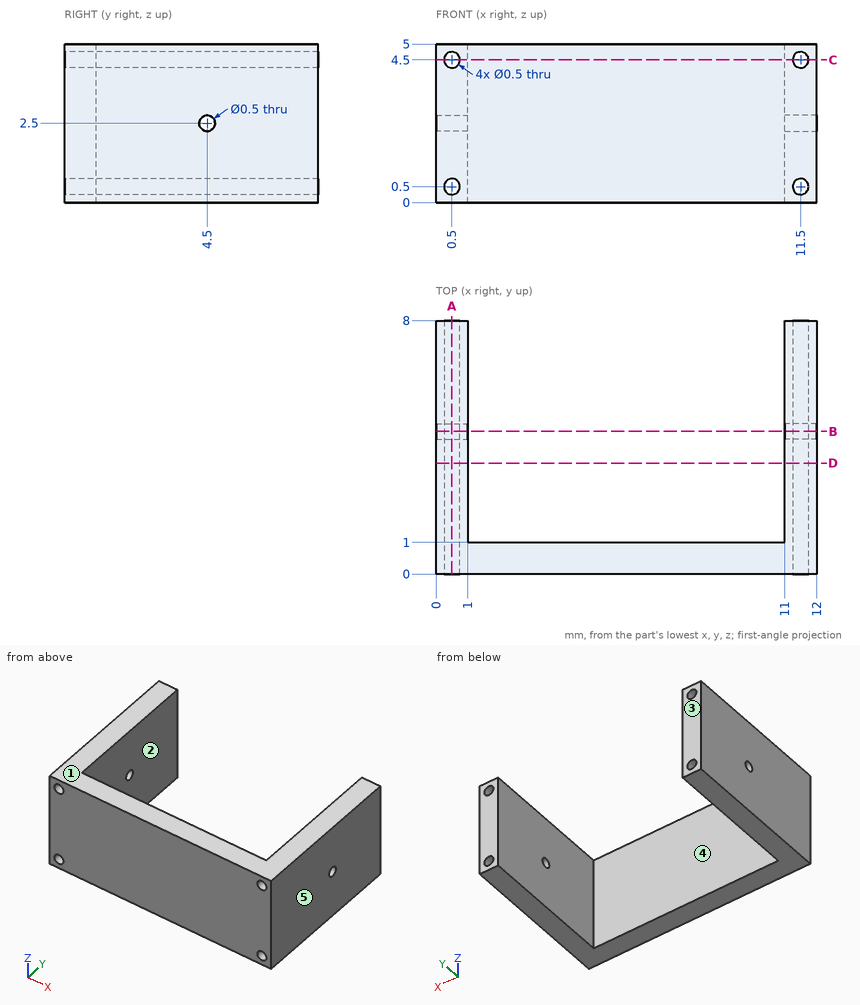
Source: three-view drawing plus pictorial views. Frame: mm from the lowest corner of the part. A direction names the side the tool comes from. Give positions to 0.01 mm unless a question says otherwise; leave off trailing zeros. Write each loop counter-clockwise with the first axis right and the second up, starting at its lowest first coordinate (ties: lowest second). Pieces come first, ordered by that corner, then holes.
(1) Cut plane D-D, the plane y = 3.5. Return loops of the section in (x, z).
(2) First-contact query: P1, Ø3, axis at x = 5, z = 3.5, coming from the +Y side. Flat tip, straight axial feed; report the tip coordinate or a pass-through.
(3) Cut plane C-C, the plane z = 4.5. Return loops of the section in (x, y), then the cut area to 3 significant figures.
(4) Cut plane A-A, the plane x = 0.5. Return loops of the section in (y, z), then the cut area to 3 significant figures.
(5) Cut plane B-B, the plane y = 4.5. Return loops of the section in (x, z), then the cut area to 3 significant figures.
(6) Access query for the marked faces 1 and 2. Directions: +Z, -Z, +X, -X, +Y, -Y. A direction counts if a zero-diameter tool reaches every point of the face in a straight line with its end or side. Return the directions, or none.
(7) Ray query, line 1 (X direction, y = 6.25, z = 2.65); line 2 (Y direction, x = 1.75, z = 4.2); line 3 (Y direction, x = 11.25, z = 2.6). Return the intervals inside material, ascending.
(8) Mould query, pull axis X, two halves, no side actions, for the marked faces 3, 4 and 5. Classes: released by +X, released by -X, zero draft, split by the parting line, or undercut.
Values follow:
1. outline: (0, 0) - (1, 0) - (1, 5) - (0, 5) - close; (11, 0) - (12, 0) - (12, 5) - (11, 5) - close; hole circle Ø0.5 at (0.5, 0.5); hole circle Ø0.5 at (0.5, 4.5); hole circle Ø0.5 at (11.5, 0.5); hole circle Ø0.5 at (11.5, 4.5)
2. P1: stops at y = 1
3. outline: (0, 0) - (0.25, 0) - (0.25, 8) - (0, 8) - close; (0.75, 0) - (11.25, 0) - (11.25, 8) - (11, 8) - (11, 1) - (1, 1) - (1, 8) - (0.75, 8) - close; (11.75, 0) - (12, 0) - (12, 8) - (11.75, 8) - close
3. area: 18.0 mm2
4. outline: (0, 0) - (8, 0) - (8, 0.25) - (0, 0.25) - close; (0, 0.75) - (8, 0.75) - (8, 4.25) - (0, 4.25) - close; (0, 4.75) - (8, 4.75) - (8, 5) - (0, 5) - close; hole circle Ø0.5 at (4.5, 2.5)
4. area: 31.8 mm2
5. outline: (0, 0) - (1, 0) - (1, 2.25) - (0, 2.25) - close; (0, 2.75) - (1, 2.75) - (1, 5) - (0, 5) - close; (11, 0) - (12, 0) - (12, 2.25) - (11, 2.25) - close; (11, 2.75) - (12, 2.75) - (12, 5) - (11, 5) - close; hole circle Ø0.5 at (0.5, 0.5); hole circle Ø0.5 at (0.5, 4.5); hole circle Ø0.5 at (11.5, 0.5); hole circle Ø0.5 at (11.5, 4.5)
5. area: 8.21 mm2
6. face 1: +Z, +X, -X, +Y, -Y
6. face 2: +Z, -Z, +Y
7. line 1: x = 0 to 1, 11 to 12
7. line 2: y = 0 to 1
7. line 3: y = 0 to 4.27, 4.73 to 8
8. face 3: zero draft
8. face 4: undercut
8. face 5: released by +X
